from build123d import *

# Parameters (mm, degrees)
SKETCH1_W                    = 34
SKETCH1_H                    = 30
SKETCH1_R                    = 10
BASE_FLANGE1_DEPTH           = 0.7366
EDGE_FLANGE1_STRIP_W         = 4.4196
EDGE_FLANGE1_STRIP_H         = 0.7366
EDGE_FLANGE1_STRIP_CUT_DEPTH = 30
EDGE_FLANGE1_DEPTH           = 30
EDGE_FLANGE2_STRIP_W         = 4.4196
EDGE_FLANGE2_STRIP_H         = 0.7366
EDGE_FLANGE2_STRIP_CUT_DEPTH = 30
EDGE_FLANGE2_DEPTH           = 30
EDGE_FLANGE2_START           = 0.7366
EDGE_FLANGE2_FLAT_DEPTH      = 0.7366
HEM1_START                   = -15
HEM1_DEPTH                   = 30
HEM1_2_DEPTH                 = 30
EDGE_FLANGE3_STRIP_W         = 4.4196
EDGE_FLANGE3_STRIP_H         = 0.7366
EDGE_FLANGE3_STRIP_CUT_DEPTH = 30
EDGE_FLANGE3_DEPTH           = 30
EDGE_FLANGE4_STRIP_W         = 4.4196
EDGE_FLANGE4_STRIP_H         = 0.7366
EDGE_FLANGE4_STRIP_CUT_DEPTH = 30
EDGE_FLANGE4_DEPTH           = 30
F_5_5_5_5_DIAMETER_HOLE1_D   = 5.5


# Read off the part's stored shape, not the designer's step: Hem1
# Sheet-metal steps are written as plain solids
with BuildPart() as part:
    # Sketch1 → Base-Flange1 (new body)
    with BuildSketch(Plane(origin=(0, 0, 0), x_dir=(1, 0, 0), z_dir=(0, 1, 0))):
        Rectangle(SKETCH1_W, SKETCH1_H)
        with Locations(Location((0, 0, 0), (0, 0, 270))):
            Circle(SKETCH1_R, mode=Mode.SUBTRACT)
    extrude(amount=-BASE_FLANGE1_DEPTH)

    # Edge-Flange1 strip (across the edge) → Edge-Flange1 strip cut (cut)
    with BuildSketch(Plane(origin=(17, 0, 15), x_dir=(-1, 0, 0), z_dir=(0, 0, -1))):
        with Locations((-1.4732, -0.3683)):
            Rectangle(EDGE_FLANGE1_STRIP_W, EDGE_FLANGE1_STRIP_H)
    extrude(amount=EDGE_FLANGE1_STRIP_CUT_DEPTH, mode=Mode.SUBTRACT)

    # Edge-Flange1 section (across the edge) → Edge-Flange1 (add)
    with BuildSketch(Plane(origin=(17, 0, 15), x_dir=(-1, 0, 0), z_dir=(0, 0, -1))):
        with BuildLine():
            Line((-0.7366, 0.7366), (-0.7366, 25))
            Line((-0.7366, 25), (0, 25))
            Line((0, 25), (0, 0.7366))
            ThreePointArc((0, 0.7366), (0.215745145, 0.215745145), (0.7366, 0))
            Line((0.7366, 0), (0.7366, -0.7366))
            ThreePointArc((0.7366, -0.7366), (-0.30510971, -0.30510971), (-0.7366, 0.7366))
        make_face()
    extrude(amount=EDGE_FLANGE1_DEPTH)

    # Edge-Flange2 strip (across the edge) → Edge-Flange2 strip cut (cut)
    with BuildSketch(Plane(origin=(-17, 0, -15), x_dir=(1, 0, 0), z_dir=(0, 0, 1))):
        with Locations((-1.4732, -0.3683)):
            Rectangle(EDGE_FLANGE2_STRIP_W, EDGE_FLANGE2_STRIP_H)
    extrude(amount=EDGE_FLANGE2_STRIP_CUT_DEPTH, mode=Mode.SUBTRACT)

    # Edge-Flange2 bend section (across the edge) → Edge-Flange2 (add)
    with BuildSketch(Plane(origin=(-17, 0, -15), x_dir=(1, 0, 0), z_dir=(0, 0, 1))):
        with BuildLine():
            Line((-0.7366, 0.7366), (0, 0.7366))
            ThreePointArc((0, 0.7366), (0.215745145, 0.215745145), (0.7366, 0))
            Line((0.7366, 0), (0.7366, -0.7366))
            ThreePointArc((0.7366, -0.7366), (-0.30510971, -0.30510971), (-0.7366, 0.7366))
        make_face()
    extrude(amount=EDGE_FLANGE2_DEPTH)

    # Edge-Flange2 profile (on flange) → Edge-Flange2 flat (add)
    with BuildSketch(Plane.ZY.offset(17).offset(EDGE_FLANGE2_START)):
        with BuildLine():
            ThreePointArc((15, 20), (0, 35), (-15, 20))
            Line((-15, 20), (-15, 0.7366))
            Line((-15, 0.7366), (15, 0.7366))
            Line((15, 0.7366), (15, 20))
        make_face()
    extrude(amount=-EDGE_FLANGE2_FLAT_DEPTH)

    # Hem1 outline → Hem1 (cut)
    with BuildSketch(Plane.XY.offset(HEM1_START)):
        with BuildLine():
            ThreePointArc((17, 24.2134), (17.212984467, 24.751642306), (17.7366, 24.998409274))
            Line((17.7366, 24.998409274), (17.7366, 25))
            Line((17.7366, 25), (17, 25))
            Line((17, 25), (17, 24.2134))
        make_face()
    extrude(amount=HEM1_DEPTH, mode=Mode.SUBTRACT)

    # Hem1 2 outline → Hem1 2 (add)
    with BuildSketch(Plane.XY.offset(HEM1_START)):
        with BuildLine():
            Line((17.8366, -0.7366), (18.5732, -0.7366))
            Line((18.5732, -0.7366), (18.5732, 24.2134))
            ThreePointArc((18.5732, 24.2134), (18.324842306, 24.787015533), (17.7366, 24.998409274))
            Line((17.7366, 24.998409274), (17.7366, 24.2134))
            ThreePointArc((17.7366, 24.2134), (17.7866, 24.2634), (17.8366, 24.2134))
            Line((17.8366, 24.2134), (17.8366, -0.7366))
        make_face()
    extrude(amount=HEM1_2_DEPTH)

    # Edge-Flange3 strip (across the edge) → Edge-Flange3 strip cut (cut)
    with BuildSketch(Plane(origin=(18.5732, -0.7366, 15), x_dir=(0, 1, 0), z_dir=(0, 0, -1))):
        with Locations((-0.7366, -0.3683)):
            Rectangle(EDGE_FLANGE3_STRIP_W, EDGE_FLANGE3_STRIP_H)
    extrude(amount=EDGE_FLANGE3_STRIP_CUT_DEPTH, mode=Mode.SUBTRACT)

    # Edge-Flange3 section (across the edge) → Edge-Flange3 (add)
    with BuildSketch(Plane(origin=(18.5732, -0.7366, 15), x_dir=(0, 1, 0), z_dir=(0, 0, -1))):
        with BuildLine():
            Line((0, 0.7366), (0, 14.2734))
            Line((0, 14.2734), (0.7366, 14.2734))
            Line((0.7366, 14.2734), (0.7366, 0.7366))
            ThreePointArc((0.7366, 0.7366), (0.952345145, 0.215745145), (1.4732, 0))
            Line((1.4732, 0), (1.4732, -0.7366))
            ThreePointArc((1.4732, -0.7366), (0.43149029, -0.30510971), (0, 0.7366))
        make_face()
    extrude(amount=EDGE_FLANGE3_DEPTH)

    # Edge-Flange4 strip (across the edge) → Edge-Flange4 strip cut (cut)
    with BuildSketch(Plane(origin=(32.8466, 0, 15), x_dir=(-1, 0, 0), z_dir=(0, 0, -1))):
        with Locations((-1.4732, -0.3683)):
            Rectangle(EDGE_FLANGE4_STRIP_W, EDGE_FLANGE4_STRIP_H)
    extrude(amount=EDGE_FLANGE4_STRIP_CUT_DEPTH, mode=Mode.SUBTRACT)

    # Edge-Flange4 section (across the edge) → Edge-Flange4 (add)
    with BuildSketch(Plane(origin=(32.8466, 0, 15), x_dir=(-1, 0, 0), z_dir=(0, 0, -1))):
        with BuildLine():
            Line((-0.7366, 0.7366), (-0.7366, 34.2634))
            Line((-0.7366, 34.2634), (0, 34.2634))
            Line((0, 34.2634), (0, 0.7366))
            ThreePointArc((0, 0.7366), (0.215745145, 0.215745145), (0.7366, 0))
            Line((0.7366, 0), (0.7366, -0.7366))
            ThreePointArc((0.7366, -0.7366), (-0.30510971, -0.30510971), (-0.7366, 0.7366))
        make_face()
    extrude(amount=EDGE_FLANGE4_DEPTH)

    # Ø5.5 (5.5) Diameter Hole1 (through all)
    with Locations(Plane.ZY.offset(17.7366)):
        with Locations((0, 20)):
            Hole(F_5_5_5_5_DIAMETER_HOLE1_D / 2)


solid = part.part
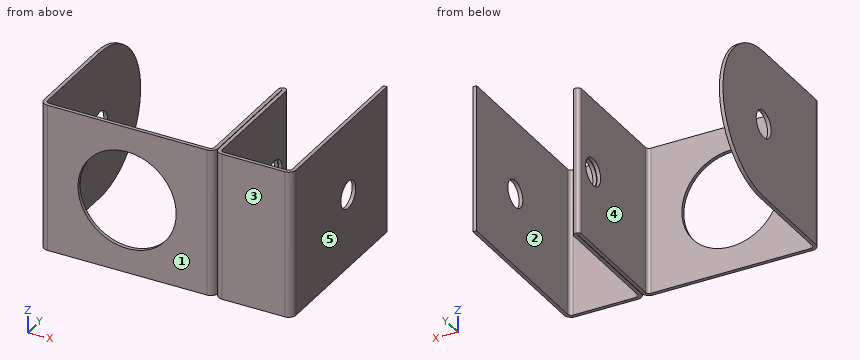
Build history of the part. All positions in model axes, mm. Face numbers are marked on the shaded views. A direction names the side the tool comes from. Coordinates: 2 decimals unless noted, no trailing zeros. Order: outer loops, then holes, each group sorted by start corner. A loop starts at its lowest first (then second) coordinate and runs counter-clockwise, first axis right, second up. Notation, with made-up numbers: (12, 21.25) -> (31, 21.25) arc R19 cw to (31, 36.25) -> close; hole circle Ø9 at (78.5, 18). An arc over 180 degrees is marked (long way). One line per item, written item: value.
(1) Mould opens along X. For the marked faces 3, 4 and 5 say: pulls with the +X half, pulls with the -X half, needs draft (parallel to the pull), parting line crosses it, or undercut.
Checked values:
face 3: needs draft
face 4: undercut
face 5: pulls with the +X half
(2) Slice it at D-D, the plane y = 28.5. List the corners of the cut face in (x, z).
Checked values:
outline: (-17.74, -12.36) -> (-17, -12.36) -> (-17, 12.36) -> (-17.74, 12.36) -> close; (32.85, -15) -> (33.58, -15) -> (33.58, 15) -> (32.85, 15) -> close
(3) Slice it at A-A, the plane x = 0. List the corners of the cut face in (y, z).
Checked values:
outline: (-0.74, -15) -> (0, -15) -> (0, -10) -> (-0.74, -10) -> close; (-0.74, 10) -> (0, 10) -> (0, 15) -> (-0.74, 15) -> close
(4) Probe line 1 (X direction, y = 29.5, z = 0.75); line 2 (Y direction, x = 5, z = -9.75); line 3 (Y direction, x = 33.45, z = 0). List the from-to ranges inside material, lowest first. Write a range as [from, to].
Checked values:
line 1: [-17.74, -17], [32.85, 33.58]
line 2: [-0.74, 0]
line 3: [0.12, 17.25], [22.75, 34.26]
(5) Slice it at C-C, the plane z = 3.75. List the corners of the cut face in (x, y).
Checked values:
outline: (-17.74, 0.74) arc R1.47 ccw to (-16.26, -0.74) -> (-9.27, -0.74) -> (-9.27, 0) -> (-16.26, 0) arc R0.74 cw to (-17, 0.74) -> (-17, 34.52) -> (-17.74, 34.52) -> close; (9.27, -0.74) -> (16.26, -0.74) arc R1.47 ccw to (17.74, 0.74) -> (17.74, 24.21) arc R0.05 cw to (17.84, 24.21) -> (17.84, 0.74) arc R1.47 ccw to (19.31, -0.74) -> (32.11, -0.74) arc R1.47 ccw to (33.58, 0.74) -> (33.58, 34.26) -> (32.85, 34.26) -> (32.85, 0.74) arc R0.74 cw to (32.11, 0) -> (19.31, 0) arc R0.74 cw to (18.57, 0.74) -> (18.57, 24.21) arc R0.79 ccw to (17, 24.21) -> (17, 0.74) arc R0.74 cw to (16.26, 0) -> (9.27, 0) -> close
(6) Tool access for the marked faces 1 and 2: list every direction of +Z, -Z, +X, -X, +Y, -Y with a clear straight run to the whole face (end or side of a thin tool).
Checked values:
face 1: +Z, -Z, +X, -X, -Y
face 2: +Z, -Z, +Y
(7) Drop flat-ended pins along their axis: pin 1 Ø14 at (x, z) = (26, 5) entering from +Y; pin 2 Ø6 at (x, z) = (-10, -8.5) entering from +Y. Give the stop position or say it passes through.
Checked values:
pin 1: y = 34.26
pin 2: y = 0
(8) Slice it at B-B, the plane y = 7.5. List the corners of the cut face in (x, z).
Checked values:
outline: (-17.74, -15) -> (-17, -15) -> (-17, 15) -> (-17.74, 15) -> close; (17, -15) -> (17.74, -15) -> (17.74, 15) -> (17, 15) -> close; (17.84, -15) -> (18.57, -15) -> (18.57, 15) -> (17.84, 15) -> close; (32.85, -15) -> (33.58, -15) -> (33.58, 15) -> (32.85, 15) -> close
